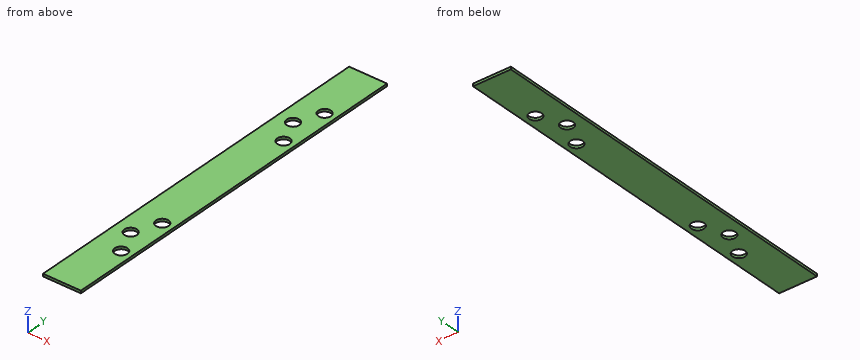
from build123d import *

# Parameters (mm, degrees)
F0_W     = 38.1
F0_H     = 378.714
F1_DEPTH = 2.54
F5_D     = 12.7
F9_D     = 12.7


with BuildPart() as f1:
    # F0 (on Top) → F1 (new body)
    with BuildSketch(Plane.XY):
        Rectangle(F0_W, F0_H)
    extrude(amount=F1_DEPTH)

    # F5 (through all)
    with Locations(Plane.XY.offset(2.54)):
        with Locations((-3.175, 100.457), (7.9375, 75.057), (7.9375, 125.857)):
            Hole(F5_D / 2)

    # F9 (through all)
    with Locations(Plane.XY.offset(2.54)):
        with Locations((7.9375, -125.857), (-3.175, -100.457), (7.9375, -75.057)):
            Hole(F9_D / 2)


solid = f1.part
Verification items for the finished model (mm, model axes). Round coordinates to 2 decimals unless told otherwise and drop trailing zeros. Order: outer loops, then holes, each group sorted by start corner. A loop starts at its lowest first (then second) coordinate and runs counter-clockwise, first axis right, second up.
1. Section check B-B on z = 1.7. State how many separate pieces and enclosed holes the cut face has, then the cut area to 3 significant figures.
Final values:
separate pieces: 1
enclosed holes: 6
area: 13,700 mm2
2. Section check A-A on x = 10. Record the cut outline in (y, z), then the cut area to 3 significant figures.
Final values:
outline: (-189.36, 0) - (-131.86, 0) - (-131.86, 2.54) - (-189.36, 2.54) - close; (-119.85, 0) - (-81.06, 0) - (-81.06, 2.54) - (-119.85, 2.54) - close; (-69.05, 0) - (69.05, 0) - (69.05, 2.54) - (-69.05, 2.54) - close; (81.06, 0) - (119.85, 0) - (119.85, 2.54) - (81.06, 2.54) - close; (131.86, 0) - (189.36, 0) - (189.36, 2.54) - (131.86, 2.54) - close
area: 840 mm2
3. Thickness scan on L1, parallel to Y at x = 7.5, z = 0.8; L2, parallel to Y at x = 5.5, z = 0.2; L3, parallel to Y at x = -6, z = 0.15. Record the ranges inside material, lowest first.
Final values:
L1: y = -189.36 to -132.19, -119.52 to -81.39, -68.72 to 68.72, 81.39 to 119.52, 132.19 to 189.36
L2: y = -189.36 to -131.72, -119.99 to -80.92, -69.19 to 69.19, 80.92 to 119.99, 131.72 to 189.36
L3: y = -189.36 to -106.14, -94.77 to 94.77, 106.14 to 189.36
